Source: CAD feature listing. Evaluate the final solid. Frame: model axes, mm. Face numbers are marked on the shaded views. A direction names the side the tool comes from. Round coordinates to 2 decimals unless told otherwise and drop trailing zeros. Loops run counter-clockwise (first coordinate to the right, second up) from the corner with the lowest first, then second, coordinate; pieces in that order, holes last. Notation, with made-up numbers: M -0.75,1.25 L 44.25,1.25 A24 cw 44.25,39.25 Z; hole C 79,12.5 d6. An arc over 180 degrees is marked long. Answer as a JSON object with one key per item and string values.
from build123d import *

# Parameters (mm, degrees)
F1_DEPTH = 10
F2_DEPTH = 15
F3_W     = 28.4455648065
F3_H     = 32.6516358182
F4_DEPTH = 50
F5_DEPTH = 45
F6_DEPTH = 3


with BuildPart() as f1:
    # F0 (on Top) → F1 (new body)
    with BuildSketch(Plane.XY):
        Polygon((17.2702856362, 36.0247381032), (-59.6364587545, 36.0247381032), (-59.6364587545, 13.3574875072), (-26.1752791703, 13.3574875072), (-26.1752791703, -19.294148311), (-59.9063038826, -19.294148311), (-59.9063038826, -40.3423085809), (17.2702856362, -40.3423085809), (17.2702856362, -19.294148311), (59.9063113332, -19.294148311), (59.9063113332, 13.3574875072), (17.2702856362, 13.3574875072), align=None)
    extrude(amount=F1_DEPTH)

    # F2 (cut): a face of the model
    f2_faces = [f1.faces().sort_by_distance(p)[0] for p in [
        (-26.1752791703, -2.9683304019, 5),
    ]]
    extrude(f2_faces, amount=-F2_DEPTH, mode=Mode.SUBTRACT)

    # F3 (on face) → F4 (join)
    with BuildSketch(Plane.XY.offset(10)):
        with Locations((3.047503233, -2.9683304019)):
            Rectangle(F3_W, F3_H)
    extrude(amount=F4_DEPTH)

    # F5 (add): a face of the model
    f5_faces = [f1.faces().sort_by_distance(p)[0] for p in [
        (3.047503233, -2.9683304019, 60),
    ]]
    extrude(f5_faces, amount=F5_DEPTH)

    # F6 (add): a face of the model
    f6_faces = [f1.faces().sort_by_distance(p)[0] for p in [
        (3.047503233, -19.294148311, 57.5),
    ]]
    extrude(f6_faces, amount=F6_DEPTH)


solid = f1.part
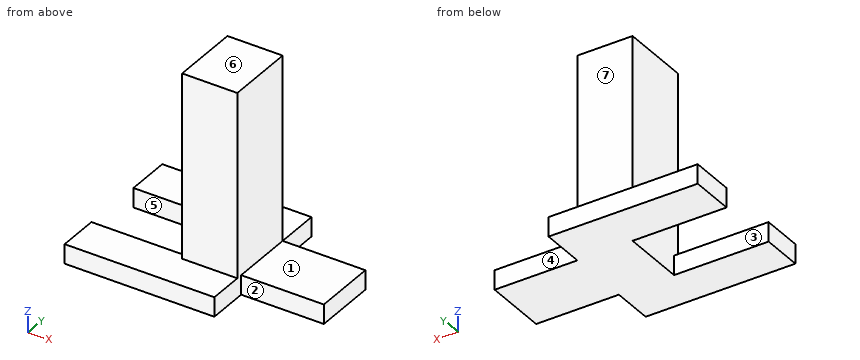
Item 1: Section C-C on z = 43.5. Return the cut outline in (x, y), then the cut area to 3 significant figures.
Answer sheet:
{"outline": "M -11.18,-22.29 L 17.27,-22.29 L 17.27,13.36 L -11.18,13.36 Z", "area": "1,010 mm²"}
Item 2: Access query for the marked faces 1, 2, 3 and 4. Directions: +Z, -Z, +X, -X, +Y, -Y. A direction counts if a zero-diameter tool reaches every point of the face in a straight line with its end or side. Return the directions, or none.
Answer sheet:
{"face 1": "+Z, +X, +Y, -Y", "face 2": "+Z, -Z, +X, -Y", "face 3": "+Z, -Z, -X", "face 4": "+Z, -Z, +X, +Y"}
Item 3: Line query: probe 1 along X at (y, z) = (-9.5, 7.5); probe 2 along Z at (x, y) = (-54, 26.5); probe 3 along Y at (x, z) = (1.5, 76.5). Output: solid intervals per line, ascending. Write a range as from..to.
Answer sheet:
{"probe 1": "x = -11.18..59.91", "probe 2": "z = 0..10", "probe 3": "y = -22.29..13.36"}
Item 4: Pull-direction query (Y, two-part tool) for the marked faces 5, 6 and 7; classes: pulls with the +Y half, pulls with the -Y half, needs draft (parallel to the pull), parting line crosses it, or undercut.
Answer sheet:
{"face 5": "undercut", "face 6": "needs draft", "face 7": "pulls with the +Y half"}
Item 5: Contact query for flat-ended pins moving along their axis: pin 1 Ø10.5 at (x, y) = (-15, -27) entering from +Z; pin 2 Ø8 at (y, z) = (20, 4) entering from +X; pin 3 Ø11 at (x, z) = (49, 4.5) entering from -Y. Output: stop coordinate, or through.
Answer sheet:
{"pin 1": "stops at z = 10", "pin 2": "stops at x = 17.27", "pin 3": "stops at y = -19.29"}
Item 6: Section D-D on y = -13. Return the cut outline in (x, z), then the cut area to 3 significant figures.
Answer sheet:
{"outline": "M -11.18,0 L 59.91,0 L 59.91,10 L 17.27,10 L 17.27,105 L -11.18,105 Z", "area": "3,410 mm²"}
Item 7: Section A-A on x = -50.5. Return the cut outline in (y, z), then the cut area to 3 significant figures.
Answer sheet:
{"outline": "M -40.34,0 L -19.29,0 L -19.29,10 L -40.34,10 Z; M 13.36,0 L 36.02,0 L 36.02,10 L 13.36,10 Z", "area": "437 mm²"}
Item 8: Section B-B on x = 11. Return the cut outline in (y, z).
Answer sheet:
{"outline": "M -40.34,0 L 36.02,0 L 36.02,10 L 13.36,10 L 13.36,105 L -22.29,105 L -22.29,10 L -40.34,10 Z"}
